```python
from build123d import *

# Parameters (mm, degrees)
BASE_FLANGE1_DEPTH         = 25.4
F_1_8_0_1250_DOWEL_HOLE1_D = 4.7625
CUT_EXTRUDE1_DEPTH         = 242.668219578
CUT_EXTRUDE1_DEPTH_BACK    = 242.668219578
SKETCH8_R                  = 2.1828125


# Sheet-metal steps are written as plain solids
with BuildPart() as part:
    # Sketch1 → Base-Flange1 (new body)
    with BuildSketch(Plane(origin=(0, 0, 0), x_dir=(1, 0, 0), z_dir=(0, 1, 0))):
        with BuildLine():
            Line((-98.425, 133.223), (-98.425, 3.175))
            ThreePointArc((-98.425, 3.175), (-97.49506403, 0.92993597), (-95.25, 0))
            Line((-95.25, 0), (95.25, 0))
            ThreePointArc((95.25, 0), (97.49506403, 0.92993597), (98.425, 3.175))
            Line((98.425, 3.175), (98.425, 133.223))
            Line((98.425, 133.223), (101.6, 133.223))
            Line((101.6, 133.223), (101.6, 3.175))
            ThreePointArc((101.6, 3.175), (99.740128061, -1.315128061), (95.25, -3.175))
            Line((95.25, -3.175), (-95.25, -3.175))
            ThreePointArc((-95.25, -3.175), (-99.740128061, -1.315128061), (-101.6, 3.175))
            Line((-101.6, 3.175), (-101.6, 133.223))
            Line((-101.6, 133.223), (-98.425, 133.223))
        make_face()
    extrude(amount=BASE_FLANGE1_DEPTH)

    # 1/8 (0.1250) Dowel Hole1 (through all)
    with Locations(Plane(origin=(0, 0, 0), x_dir=(-1, 0, 0), z_dir=(0, 0, -1))):
        with Locations((76.2, 12.7), (-76.2, 12.7)):
            Hole(F_1_8_0_1250_DOWEL_HOLE1_D / 2)

    # Sketch8 → Cut-Extrude1 (cut, two sides: drawn at the far end of the back side and taken through both)
    with BuildSketch(Plane.ZY.offset(-98.425).offset(-CUT_EXTRUDE1_DEPTH_BACK)):
        with Locations((-57.785, 12.7)):
            Circle(SKETCH8_R)
        with Locations((-123.063, 12.7)):
            Circle(SKETCH8_R)
    extrude(amount=CUT_EXTRUDE1_DEPTH + CUT_EXTRUDE1_DEPTH_BACK, mode=Mode.SUBTRACT)


solid = part.part
```
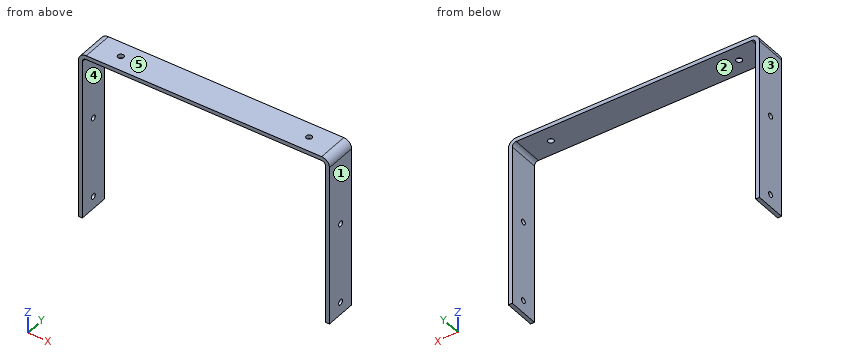
Source: CAD feature listing. Evaluate the final solid. Frame: model axes, mm. Face numbers are marked on the shaded views. A direction names the side the tool comes from. Round coordinates to 2 decimals unless told otherwise and drop trailing zeros. Loops run counter-clockwise (first coordinate to the right, second up) from the corner with the lowest first, then second, coordinate; pieces in that order, holes last.
1. Contact query for flat-ended pins moving along their axis: pin 1 (10 mm diameter, centred on x = 9.5, y = 18.5, fed in from -Z); pin 2 (5.5 mm diameter, centred on x = -76.2, y = 12.7, fed in from +Z) (3 decimals); pin 3 (4 mm diameter, centred on y = 12.7, z = -123.063, fed in from -X). Output: stop coordinate, or through.
2. Access query for the marked faces 1 and 2. Directions: +Z, -Z, +X, -X, +Y, -Y. A direction counts if a zero-diameter tool reaches every point of the face in a straight line with its end or side. Return the directions, or none.
3. Mould query, pull axis X, two halves, no side actions, for the marked faces 3, 4 and 5. Classes: released by +X, released by -X, zero draft, split by the parting line, or undercut.
4. Section query C-C on x = -76.2. Output: boundary loops of the cut face in (y, z) (3 decimals), and give its area (3 significant figures).
5. Section query B-B on z = -91. Output: boundary loops of the cut face in (x, y) (3 decimals).
6. Section query A-A on y = 19.5. Output: boundary loops of the cut face in (x, z) (3 decimals), and give its area (3 significant figures).
7. Section query D-D on x = -16. Output: boundary loops of the cut face in (y, z) (3 decimals).
8. Ray query, L1, parallel to X at y = 16.5, z = -54.5 (3 decimals); L2, parallel to Z at x = -99.1, y = 12.7; L3, parallel to Z at x = -99.3, y = 12.7. Return the intervals inside material, ascending.
Answers below:
1. pin 1: stops at z = 0
1. pin 2: stops at z = 3.175
1. pin 3: passes through
2. face 1: +Z, -Z, +X, +Y, -Y
2. face 2: -Z, +Y, -Y
3. face 3: released by -X
3. face 4: undercut
3. face 5: zero draft
4. outline: (0, 0) - (10.319, 0) - (10.319, 3.175) - (0, 3.175) - close; (15.081, 0) - (25.4, 0) - (25.4, 3.175) - (15.081, 3.175) - close
4. area: 65.5 mm2
5. outline: (-101.6, 0) - (-98.425, 0) - (-98.425, 25.4) - (-101.6, 25.4) - close; (98.425, 0) - (101.6, 0) - (101.6, 25.4) - (98.425, 25.4) - close
6. outline: (-101.6, -133.223) - (-98.425, -133.223) - (-98.425, -3.175) arc R3.175 cw to (-95.25, 0) - (95.25, 0) arc R3.175 cw to (98.425, -3.175) - (98.425, -133.223) - (101.6, -133.223) - (101.6, -3.175) arc R6.35 ccw to (95.25, 3.175) - (-95.25, 3.175) arc R6.35 ccw to (-101.6, -3.175) - close
6. area: 1,480 mm2
7. outline: (0, 0) - (25.4, 0) - (25.4, 3.175) - (0, 3.175) - close
8. L1: x = -101.6 to -98.425, 98.425 to 101.6
8. L2: z = -133.22 to -125.25, -120.88 to -59.97, -55.6 to 1.87
8. L3: z = -133.22 to -125.25, -120.88 to -59.97, -55.6 to 1.72
